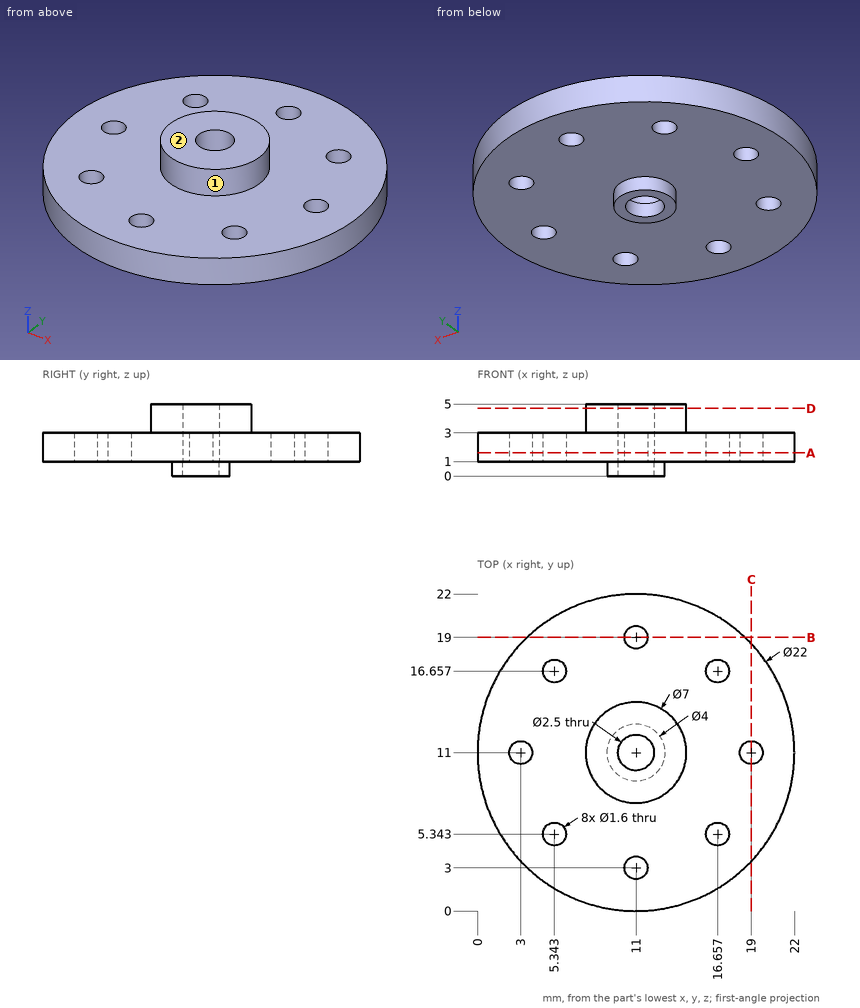
Part print with two shaded views. Sizes in mm from the minimum x, y, z corner. A direction names the side the tool comes from. Round coordinates to 2 decimals unless told otherwise and drop trailing zeros. Order: outer loops, then holes, each group sorted by start corner. A loop starts at its lowest first (then second) coordinate and runs counter-clockwise, first axis right, second up. Notation, with made-up numbers: M 43,68.25 L 101,68.25 A28 ccw 101,106.25 Z; hole C -16,-17.5 d4. An arc over 180 degrees is marked long. Answer in a Markdown table with one row per item. Add a question column.
Q1. Wall check: L1, parallel to Y at x = 11, z = 1.5; L2, parallel to X at y = 17, z = 1.2; L3, parallel to Y at x = 16.25, z = 1.2. Give the ranges that are in metal, low to high. Write a range as from..to.
Q2. Cut at B-B on y = 19. Give the cut face in (x, z), and give its area (3 significant figures).
Q3. 3-axis set-ups, long thin cutter, end or side, ignore diameter. For the marked faces 1 and 2: which of +Z, -Z, +X, -X, +Y, -Y reach the whole face in a straight line?
Q4. Cut at A-A on z = 1.6. Give the number of separate pieces and of enclosed holes in the cut face, and give its area (3 significant figures).
Q5. Pin check, flat tips, straight feed: pin 1 (10 mm diameter, centred on x = 4, y = 14.5, fed in from -Z); pin 2 (1.8 mm diameter, centred on x = 5.34, y = 5.34, fed in from +Z); pin 3 (11 mm diameter, centred on x = 15, y = 15.5, fed in from -Z); pin 4 (3 mm diameter, centred on y = 17.5, z = 1.5, fed in from +X). Stop position of each tip, or through.
Q6. Cut at D-D on z = 4.7. Give the cut face in (x, y).
Established:
| question | item | result |
|---|---|---|
| 1 | L1 | y = 0..2.2, 3.8..9.75, 12.25..18.2, 19.8..22 |
| 1 | L2 | x = 1.78..4.62, 6.07..15.93, 17.38..20.22 |
| 1 | L3 | y = 1.33..4.65, 6.03..15.97, 17.35..20.67 |
| 2 | outline | M 3.45,1 L 10.2,1 L 10.2,3 L 3.45,3 Z; M 11.8,1 L 18.55,1 L 18.55,3 L 11.8,3 Z |
| 2 | area | 27.0 mm2 |
| 3 | face 1 | +Z |
| 3 | face 2 | +Z, +X, -X, +Y, -Y |
| 4 | separate pieces | 1 |
| 4 | enclosed holes | 9 |
| 4 | area | 359 mm2 |
| 5 | pin 1 | stops at z = 1 |
| 5 | pin 2 | stops at z = 3 |
| 5 | pin 3 | stops at z = 0 |
| 5 | pin 4 | stops at x = 20.8 |
| 6 | outline | C 11,11 d7; hole C 11,11 d2.5 |
